The model under review builds one solid part; all positions refer to its coordinate system, in mm. A direction names the side the tool comes from. Round coordinates to 2 decimals unless told otherwise and drop trailing zeros. Loops run counter-clockwise (first coordinate to the right, second up) from the corner with the lowest first, then second, coordinate; pieces in that order, holes last. Notation, with made-up numbers: M -28.5,18 L -15.5,18 A4 ccw -15.5,22 Z; hole C 10.5,65 d7. An arc over 180 degrees is marked long. Use a Markdown table: item, result. Add a question column.
```python
from build123d import *

# Parameters (mm, degrees)
SKETCH1_W            = 48
SKETCH1_H            = 53
BOSS_EXTRUDE1_DEPTH  = 10
SKETCH2_W            = 48
SKETCH2_H            = 5.616325
BOSS_EXTRUDE2_DEPTH  = 33.1917878
SKETCH4_W            = 4
SKETCH4_H            = 10
BOSS_EXTRUDE4_DEPTH  = 40
SKETCH5_W            = 48
SKETCH5_H            = 10.8609375
BOSS_EXTRUDE5_DEPTH  = 23.1917878
SKETCH6_W            = 48
SKETCH6_H            = 5
BOSS_EXTRUDE6_DEPTH  = 42.3
SKETCH7_W            = 12.8082122
SKETCH7_H            = 16.4772625
BOSS_EXTRUDE7_DEPTH  = 48
CUT_EXTRUDE1_REACH   = 84.426
SKETCH8_R            = 11.5
SKETCH8_R_2          = 2
FILLET1_R            = 10
FILLET2_R            = 4
SKETCH9_W            = 5
SKETCH9_H            = 16.4772625
BOSS_EXTRUDE9_DEPTH  = 48
CUT_EXTRUDE2_DEPTH   = 6
SKETCH11_R           = 1.9304
CUT_EXTRUDE3_DEPTH   = 6
BOSS_EXTRUDE11_DEPTH = 3
SKETCH14_W           = 146.253560905
SKETCH14_H           = 143.633383104
SKETCH14_W_2         = 45
SKETCH14_H_2         = 17
CUT_EXTRUDE5_DEPTH   = 90.10667764
SKETCH15_W           = 68.343124148
SKETCH15_H           = 38.24816948
CUT_EXTRUDE6_DEPTH   = 44


with BuildPart() as part:
    # Sketch1 → Boss-Extrude1 (new body)
    with BuildSketch(Plane.XY):
        with Locations((24, 26.5)):
            Rectangle(SKETCH1_W, SKETCH1_H)
    extrude(amount=BOSS_EXTRUDE1_DEPTH)

    # Sketch2 → Boss-Extrude2 (add)
    with BuildSketch(Plane(origin=(0, 0, 0), x_dir=(-1, 0, 0), z_dir=(0, 0, -1))):
        with Locations((-24, -2.8081625)):
            Rectangle(SKETCH2_W, SKETCH2_H)
    extrude(amount=-BOSS_EXTRUDE2_DEPTH)

    # Sketch4 → Boss-Extrude4 (add)
    with BuildSketch(Plane.XY.offset(10)):
        with Locations((2, 48)):
            Rectangle(SKETCH4_W, SKETCH4_H)
        with Locations((46, 48)):
            Rectangle(SKETCH4_W, SKETCH4_H)
    extrude(amount=BOSS_EXTRUDE4_DEPTH)

    # Sketch5 → Boss-Extrude5 (add)
    with BuildSketch(Plane.XY.offset(10)):
        with Locations((24, 5.43046875)):
            Rectangle(SKETCH5_W, SKETCH5_H)
    extrude(amount=BOSS_EXTRUDE5_DEPTH)

    # Sketch6 → Boss-Extrude6 (add)
    with BuildSketch(Plane.XZ.offset(5.616325)):
        with Locations((24, 30.6917878)):
            Rectangle(SKETCH6_W, SKETCH6_H)
    extrude(amount=BOSS_EXTRUDE6_DEPTH)

    # Sketch7 → Boss-Extrude7 (add)
    with BuildSketch(Plane.ZY):
        with Locations((-6.4041061, 2.62230625)):
            Rectangle(SKETCH7_W, SKETCH7_H)
    extrude(amount=-BOSS_EXTRUDE7_DEPTH)

    # Sketch8 → Cut-Extrude1 (cut, up to next)
    with BuildSketch(Plane(origin=(0, 0, 28.1917878), x_dir=(-1, 0, 0), z_dir=(0, 0, -1)), mode=Mode.PRIVATE) as cut_extrude1_sk1:
        with Locations((-24, -26.616325)):
            Circle(SKETCH8_R)
    cut_extrude1_tool1 = extrude(cut_extrude1_sk1.sketch, amount=-CUT_EXTRUDE1_REACH, mode=Mode.PRIVATE) & part.part
    # Sketch8 → Cut-Extrude1 (cut, up to next)
    with BuildSketch(Plane(origin=(0, 0, 28.1917878), x_dir=(-1, 0, 0), z_dir=(0, 0, -1)), mode=Mode.PRIVATE) as cut_extrude1_sk2:
        with Locations((-39.5, -11.116325)):
            Circle(SKETCH8_R_2)
    cut_extrude1_tool2 = extrude(cut_extrude1_sk2.sketch, amount=-CUT_EXTRUDE1_REACH, mode=Mode.PRIVATE) & part.part
    # Sketch8 → Cut-Extrude1 (cut, up to next)
    with BuildSketch(Plane(origin=(0, 0, 28.1917878), x_dir=(-1, 0, 0), z_dir=(0, 0, -1)), mode=Mode.PRIVATE) as cut_extrude1_sk3:
        with Locations((-39.5, -42.116325)):
            Circle(SKETCH8_R_2)
    cut_extrude1_tool3 = extrude(cut_extrude1_sk3.sketch, amount=-CUT_EXTRUDE1_REACH, mode=Mode.PRIVATE) & part.part
    # Sketch8 → Cut-Extrude1 (cut, up to next)
    with BuildSketch(Plane(origin=(0, 0, 28.1917878), x_dir=(-1, 0, 0), z_dir=(0, 0, -1)), mode=Mode.PRIVATE) as cut_extrude1_sk4:
        with Locations((-8.5, -11.116325)):
            Circle(SKETCH8_R_2)
    cut_extrude1_tool4 = extrude(cut_extrude1_sk4.sketch, amount=-CUT_EXTRUDE1_REACH, mode=Mode.PRIVATE) & part.part
    # Sketch8 → Cut-Extrude1 (cut, up to next)
    with BuildSketch(Plane(origin=(0, 0, 28.1917878), x_dir=(-1, 0, 0), z_dir=(0, 0, -1)), mode=Mode.PRIVATE) as cut_extrude1_sk5:
        with Locations((-8.5, -42.116325)):
            Circle(SKETCH8_R_2)
    cut_extrude1_tool5 = extrude(cut_extrude1_sk5.sketch, amount=-CUT_EXTRUDE1_REACH, mode=Mode.PRIVATE) & part.part
    add(cut_extrude1_tool1.solids().sort_by_distance((24, -26.616325, 28.191788))[0], mode=Mode.SUBTRACT)
    add(cut_extrude1_tool2.solids().sort_by_distance((39.5, -11.116325, 28.191788))[0], mode=Mode.SUBTRACT)
    add(cut_extrude1_tool3.solids().sort_by_distance((39.5, -42.116325, 28.191788))[0], mode=Mode.SUBTRACT)
    add(cut_extrude1_tool4.solids().sort_by_distance((8.5, -11.116325, 28.191788))[0], mode=Mode.SUBTRACT)
    add(cut_extrude1_tool5.solids().sort_by_distance((8.5, -42.116325, 28.191788))[0], mode=Mode.SUBTRACT)

    # Fillet1
    fillet1_edges = [part.edges().sort_by_distance(p)[0] for p in [
        (24, 10.8609375, 0),
    ]]
    fillet(fillet1_edges, radius=FILLET1_R)

    # Fillet2
    fillet2_edges = [part.edges().sort_by_distance(p)[0] for p in [
        (2, 43, 10),
        (46, 43, 10),
    ]]
    fillet(fillet2_edges, radius=FILLET2_R)

    # Sketch9 → Boss-Extrude9 (add)
    with BuildSketch(Plane(origin=(48, 0, 0), x_dir=(0, 0, -1), z_dir=(1, 0, 0))):
        with Locations((15.3082122, 2.62230625)):
            Rectangle(SKETCH9_W, SKETCH9_H)
    extrude(amount=-BOSS_EXTRUDE9_DEPTH)

    # Sketch10 → Cut-Extrude2 (cut)
    with BuildSketch(Plane.XY.offset(10)):
        Polygon((12.429, 36.979734073), (9, 38.959468146), (5.571, 36.979734073), (5.571, 33.020265927), (9, 31.040531854), (12.429, 33.020265927), align=None)
        Polygon((35.571, 36.979734073), (35.571, 33.020265927), (39, 31.040531854), (42.429, 33.020265927), (42.429, 36.979734073), (39, 38.959468146), align=None)
    extrude(amount=-CUT_EXTRUDE2_DEPTH, mode=Mode.SUBTRACT)

    # Sketch11 → Cut-Extrude3 (cut)
    with BuildSketch(Plane.XY.offset(4)):
        with Locations((9, 35)):
            Circle(SKETCH11_R)
        with Locations((39, 35)):
            Circle(SKETCH11_R)
    extrude(amount=-CUT_EXTRUDE3_DEPTH, mode=Mode.SUBTRACT)

    # Sketch12 → Boss-Extrude11 (add)
    with BuildSketch(Plane(origin=(0, 53, 0), x_dir=(1, 0, 0), z_dir=(0, 1, 0))):
        Polygon((0, 0), (0, -50), (4, -50), (4, -10), (44, -10), (44, -50), (48, -50), (48, 0), align=None)
    extrude(amount=BOSS_EXTRUDE11_DEPTH)

    # Sketch14 → Cut-Extrude5 (cut, through all)
    with BuildSketch(Plane.ZY):
        with Locations((21.574447485, 12.73606384)):
            Rectangle(SKETCH14_W, SKETCH14_H)
        with Locations((27.5, 47.5)):
            Rectangle(SKETCH14_W_2, SKETCH14_H_2, mode=Mode.SUBTRACT)
    extrude(amount=-CUT_EXTRUDE5_DEPTH, mode=Mode.SUBTRACT)

    # Sketch15 → Cut-Extrude6 (cut)
    with BuildSketch(Plane(origin=(48, 0, 0), x_dir=(0, 0, -1), z_dir=(1, 0, 0))):
        with Locations((-31.986382943, 43.740124775)):
            Rectangle(SKETCH15_W, SKETCH15_H)
    extrude(amount=-CUT_EXTRUDE6_DEPTH, mode=Mode.SUBTRACT)


solid = part.part
```
(1) For faces 1 (the face through (2, 43, 32)), 2 (the face through (0, 49, 27)), list the 3-axis set-ups (+Z, -Z, +X, -X, +Y, -Y) from which the entire face can be reached by the end or side of a thin tool; tool diameter is ignored.
(2) Insertion check: pin 1 Ø2 at (x, z) = (1.5, 34) entering from -Y. The pin has a flat end and moves straight along its axis. Give the tip position at first contact, or say it passes through.
(3) Consider section B-B, the plane z = 41. Give the boundary of the cut face in (x, y).
(4) Consider section A-A, the plane x = 2.95. Give the boundary of the cut face in (y, z), then the cut area to 3 significant figures.
(5) To check wall thickness, follow probe 1 along Y at (x, z) = (2.95, 24). State the ranges of the line that lie inside material, in increasing order.
Found:
| question | item | result |
|---|---|---|
| 1 | face 1 | +Z, +X, -X, -Y |
| 1 | face 2 | +Z, -Z, -X, +Y, -Y |
| 2 | pin 1 | stops at y = 43 |
| 3 | outline | M 0,43 L 4,43 L 4,56 L 0,56 Z |
| 4 | outline | M 39,5 L 56,5 L 56,50 L 43,50 L 43,14 A4 cw 39,10 Z |
| 4 | area | 608 mm^2 |
| 5 | probe 1 | y = 43 to 56 |
